For this review, take the finished solid that the model builds, in its own axes (mm). Coordinates: 2 decimals unless noted, no trailing zeros. Loops run counter-clockwise (first coordinate to the right, second up) from the corner with the lowest first, then second, coordinate; pieces in that order, holes last.
1. Take a section at B-B, the plane y = -19. State the section outline as (x, z) points.
2. Clearance check with flat-ended pins moving along their axes: P1, Ø1, axis at x = 14, y = -11.5, coming from the -Z side; P2, Ø1.5, axis at x = -16, z = 1, coming from the +Y side. State where each tip first meets the part, or that it passes through.
3. To check wall thickness, follow probe 1 along Y at (x, z) = (-4.5, 0.6); probe 2 along Y at (x, z) = (-5, 1.75); probe 3 along X at (y, z) = (20, 1.3). State the ranges of each line that lie inside material, in increasing order.
4. Take a section at C-C, the plane x = 9. State the section outline as (y, z) points, then the cut area to 3 significant figures.
5. Take a section at A-A, the plane z = 1.4. State the section outline as (x, y) points (3 decimals).
Autodesk Inventor part; units mm, degrees
ref_plane "YZ Plane" through (0, 0, 0) normal (1, 0, 0) x (0, 1, 0)
ref_plane "XZ Plane" through (0, 0, 0) normal (0, 1, 0) x (-1, 0, 0)
ref_plane "XY Plane" through (0, 0, 0) normal (0, 0, 1) x (1, 0, 0)
sketch "Sketch1" plane through (0, 0, 0) normal (0, 0, 1) x (1, 0, 0)
  circle A0 centre (0, 0) radius 27.5
  dimension "d0" = 55
extrude "Extrusion1" add sketch "Sketch1" along normal blind 3
sketch "Sketch2" plane through (0, 0, 0) normal (0, 0, -1) x (-1, 0, 0)
  circle A0 centre (-4.1302, 11.7979) radius 1.5 construction
  circle A1 centre (4.1302, -11.7979) radius 1.5 construction
  line L0 (-2.0593, 14.2051) -> (-1.0101, 11.208)
  line L1 (-1.0101, 11.208) -> (-3.081, 8.8009)
  line L2 (-3.081, 8.8009) -> (-6.2011, 9.3908)
  line L3 (-6.2011, 9.3908) -> (-7.2504, 12.3878)
  line L4 (-7.2504, 12.3878) -> (-5.1794, 14.795)
  line L5 (-5.1794, 14.795) -> (-2.0593, 14.2051)
  line L6 (6.2011, -9.3908) -> (7.2504, -12.3878)
  line L7 (7.2504, -12.3878) -> (5.1794, -14.795)
  line L8 (5.1794, -14.795) -> (2.0593, -14.2051)
  line L9 (2.0593, -14.2051) -> (1.0101, -11.208)
  line L10 (1.0101, -11.208) -> (3.081, -8.8009)
  line L11 (3.081, -8.8009) -> (6.2011, -9.3908)
  dimension "d7" = 5.5
  dimension "d8" = 5.5
extrude "Extrusion2" cut sketch "Sketch2" against normal up to next
equation "\"d8\" = d7"
properties part number "BottomHolder"
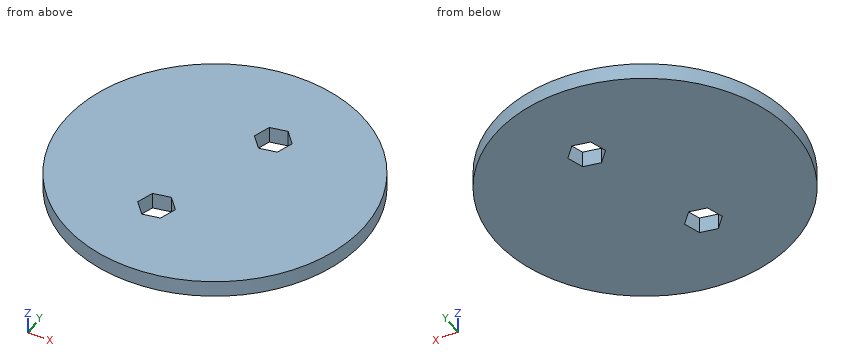
Results list:
1. outline: (-19.88, 0) - (19.88, 0) - (19.88, 3) - (-19.88, 3) - close
2. P1: stops at z = 0
2. P2: stops at y = 22.88
3. probe 1: y = -27.13 to -14.67, -9.07 to 27.13
3. probe 2: y = -27.04 to -14.76, -9.16 to 27.04
3. probe 3: x = -18.87 to 18.87
4. outline: (-25.99, 0) - (25.99, 0) - (25.99, 3) - (-25.99, 3) - close
4. area: 156 mm2
5. outline: circle Ø55 at (0, 0); hole (-7.25, -12.388) - (-5.179, -14.795) - (-2.059, -14.205) - (-1.01, -11.208) - (-3.081, -8.801) - (-6.201, -9.391) - close; hole (1.01, 11.208) - (3.081, 8.801) - (6.201, 9.391) - (7.25, 12.388) - (5.179, 14.795) - (2.059, 14.205) - close
